Geometry check sheet. Reference: the model listing, model coordinates, mm. Face numbers are marked on the shaded views. Coordinates: 2 decimals unless noted, no trailing zeros. Order: outer loops, then holes, each group sorted by start corner. A loop starts at its lowest first (then second) coordinate and runs counter-clockwise, first axis right, second up. Notation, with made-up numbers: (13, 43.25) - (57, 43.25) arc R22 cw to (57, 55.25) - close; hole circle Ø7 at (-20.75, 23.5). An arc over 180 degrees is marked (long way). Return JSON: item names as keys, results as strings. Group by question number.
Item 1: Gauge pin test, flat end, axial feed: pin 1 (3 mm diameter, centred on x = -4, z = 5.5, fed in from -Y). Record the tip position at first contact, or that the pin passes through.
Item 2: Section check C-C on y = 2. Enter the section's corners in (x, z), then the cut area to 3 significant figures.
Item 3: Scan lines: probe 1 along Z at (x, y) = (-6.5, 0.95); probe 2 along Z at (x, y) = (-8, 2.05); probe 3 along X at (y, z) = (2.6, 2). Record each from-to range of solid material in increasing order.
Item 4: Section check A-A on x = -7.75. Enter the section's corners in (y, z), then the cut area to 3 significant figures.
Item 5: Draft check along X on the marked faces 1, 2, 3 and 4. Enter one of: pulls with the +X half, pulls with the -X half, needs draft (parallel to the pull), parting line crosses it, or undercut.
Item 6: Section check B-B on z = 4.5. Enter the section's corners in (x, y), then the cut area to 3 significant figures.
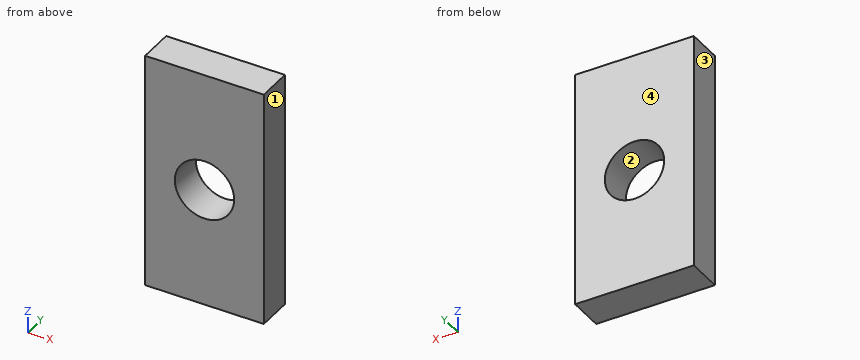
from build123d import *

# Parameters (mm, degrees)
SKETCH_1_W      = 10
SKETCH_1_H      = 20
SKETCH_1_R      = 2.5
EXTRUDE_1_DEPTH = 3


with BuildPart() as part:
    # 草圖1 → 填料-伸長1 (new body)
    with BuildSketch(Plane(origin=(0, 0, 0), x_dir=(1, 0, 0), z_dir=(0, 1, 0))):
        with Locations((-5.91954023, -3.390804598)):
            Rectangle(SKETCH_1_W, SKETCH_1_H)
        with Locations(Location((-5.91954023, -3.390804598, 0), (0, 0, 270))):
            Circle(SKETCH_1_R, mode=Mode.SUBTRACT)
    extrude(amount=EXTRUDE_1_DEPTH)


solid = part.part
Computed:
{
 "1": {"pin 1": "stops at y = 0"},
 "2": {"outline": "(-10.92, -6.61) - (-0.92, -6.61) - (-0.92, 13.39) - (-10.92, 13.39) - close; hole circle Ø5 at (-5.92, 3.39)", "area": "180 mm²"},
 "3": {"probe 1": "z = -6.61 to 0.96, 5.82 to 13.39", "probe 2": "z = -6.61 to 2, 4.78 to 13.39", "probe 3": "x = -10.92 to -8, -3.84 to -0.92"},
 "4": {"outline": "(0, -6.61) - (3, -6.61) - (3, 1.69) - (0, 1.69) - close; (0, 5.09) - (3, 5.09) - (3, 13.39) - (0, 13.39) - close", "area": "49.8 mm²"},
 "5": {"face 1": "pulls with the +X half", "face 2": "undercut", "face 3": "pulls with the -X half", "face 4": "needs draft"},
 "6": {"outline": "(-10.92, 0) - (-8.16, 0) - (-8.16, 3) - (-10.92, 3) - close; (-3.68, 0) - (-0.92, 0) - (-0.92, 3) - (-3.68, 3) - close", "area": "16.6 mm²"}
}
